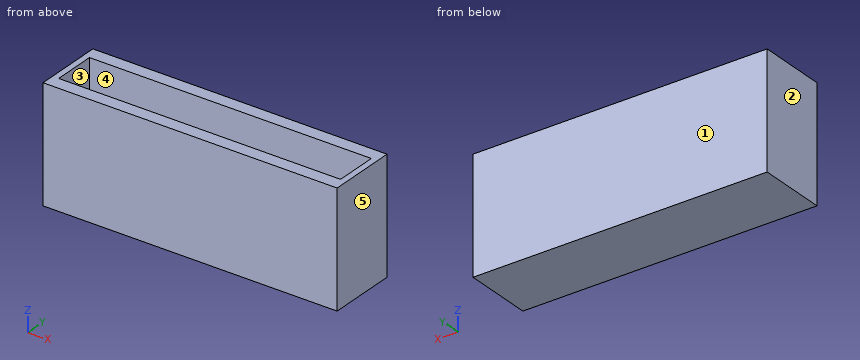
from build123d import *

# Parameters (mm, degrees)
SKETCH1_W           = 12.85
SKETCH1_H           = 5
BOSS_EXTRUDE1_DEPTH = 1.5
SKETCH3_W           = 12.31491511
SKETCH3_H           = 1.85
CUT_EXTRUDE1_DEPTH  = 3.5


with BuildPart() as part:
    # Sketch1 → Boss-Extrude1 (new body, symmetric)
    with BuildSketch(Plane(origin=(0, 0, 0), x_dir=(1, 0, 0), z_dir=(0, 1, 0))):
        Rectangle(SKETCH1_W, SKETCH1_H)
    extrude(amount=BOSS_EXTRUDE1_DEPTH, both=True)

    # Sketch3 → Cut-Extrude1 (cut)
    with BuildSketch(Plane.XY.offset(2.5)):
        Rectangle(SKETCH3_W, SKETCH3_H)
    extrude(amount=-CUT_EXTRUDE1_DEPTH, mode=Mode.SUBTRACT)


solid = part.part
Check sheet for the modelled part. Datum: model origin and axes. Units: mm. Face numbers are marked on the shaded views. A direction names the side the tool comes from. Round coordinates to 2 decimals unless told otherwise and drop trailing zeros. Loops run counter-clockwise (first coordinate to the right, second up) from the corner with the lowest first, then second, coordinate; pieces in that order, holes last.
1. Sectioned sample at A-A on x = 0.5. Record the boundary of the cut face in (y, z) (3 decimals), and give its area (4 significant figures).
2. Scan lines: probe 1 along X at (y, z) = (-0.1, -0.2) (3 decimals); probe 2 along Y at (x, z) = (-3, -0.85) (3 decimals); probe 3 along Z at (x, y) = (-3.5, -0.8). Record each from-to range of solid material in increasing order.
3. Mould release check, pull along Y, two halves, no side actions. Record for the marked faces 1, 2 and 3: released by +Y, released by -Y, zero draft, split by the parting line, or undercut.
4. Sectioned sample at B-B on z = 1.9. Record the boundary of the cut face in (x, y) (3 decimals).
5. Gauge pin test, flat end, axial feed: pin 1 Ø0.9 at (x, y) = (0, 0) entering from +Z. Record the tip position at first contact, or that the pin passes through.
6. Set-up check for the marked faces 4 and 5: record each of +Z, -Z, +X, -X, +Y, -Y from which the full face is reachable in a straight line by a thin tool's end or side.
7. Sectioned sample at C-C on y = -0.3. Record the boundary of the cut face in (x, z) (3 decimals).
Recorded:
1. outline: (-1.5, -2.5) - (1.5, -2.5) - (1.5, 2.5) - (0.925, 2.5) - (0.925, -1) - (-0.925, -1) - (-0.925, 2.5) - (-1.5, 2.5) - close
1. area: 8.525 mm2
2. probe 1: x = -6.425 to -6.157, 6.157 to 6.425
2. probe 2: y = -1.5 to -0.925, 0.925 to 1.5
2. probe 3: z = -2.5 to -1
3. face 1: released by +Y
3. face 2: zero draft
3. face 3: undercut
4. outline: (-6.425, -1.5) - (6.425, -1.5) - (6.425, 1.5) - (-6.425, 1.5) - close; hole (-6.157, -0.925) - (6.157, -0.925) - (6.157, 0.925) - (-6.157, 0.925) - close
5. pin 1: stops at z = -1
6. face 4: +Z
6. face 5: +Z, -Z, +X, +Y, -Y
7. outline: (-6.425, -2.5) - (6.425, -2.5) - (6.425, 2.5) - (6.157, 2.5) - (6.157, -1) - (-6.157, -1) - (-6.157, 2.5) - (-6.425, 2.5) - close
